Build history of the part. All positions in model axes, mm. A direction names the side the tool comes from. Coordinates: 2 decimals unless noted, no trailing zeros. Loops run counter-clockwise (first coordinate to the right, second up) from the corner with the lowest first, then second, coordinate; pieces in that order, holes last.
(1) Slice it at A-A (x = 0). Give the cut face in (y, z), and give its area (3 significant figures).
(2) Flat gauge pins, fed straight in: P1, Ø3, axis at y = 18, z = 8.5, coming from the -X side; P2, Ø18.5, axis at x = 0, y = 0, coming from the +Z side; P3, Ø7, axis at x = 0, y = -2.5, coming from the -Z side; P4, Ø8, axis at x = 0.5, y = 25, coming from the -Z side. Where does each tip first touch, or does it go through?
(3) Two-plate mould, pull along Y, no slides. Class faces 3 (the face through (-4.686, 35.694, 31.552)), 4 (the face through (7.8, -34.5, 64)), 5 (the face through (1.5, 11.4, 1.2)): pulls with the +Y half, pulls with the -Y half, needs draft (parallel to the pull), parting line crosses it, or undercut.
(4) Tool access for faces 1 (the face through (0, 0, 2.5)), 2 (the face through (-9, 9, 0)): list every direction of +Z, -Z, +X, -X, +Y, -Y with a clear straight run to the whole face (end or side of a thin tool).
(5) Slice it at D-D (z = 21). Give the cut face in (x, y), and give its area (3 significant figures).
(6) Wall check: L1, parallel to Y at x = 0, z = 1.65; L2, parallel to Y at x = 4, z = 49; L3, parallel to Y at x = -1, z = 26.5. Give the ranges that are in metal, low to high.
(7) Slice it at C-C (z = 52). Give the cut face in (x, y), and give its area (3 significant figures).
from build123d import *

# Parameters (mm, degrees)
SKETCH2_R           = 36
BOSS_EXTRUDE1_DEPTH = 74
CUT_REVOLVE1_ANGLE  = 180
CUT_EXTRUDE1_REACH  = 12
SKETCH5_W           = 97.630906447
SKETCH5_H           = 85.301230118
SKETCH6_R           = 11.5
CUT_EXTRUDE2_DEPTH  = 2.5


with BuildPart() as part:
    # Sketch2 → Boss-Extrude1 (new body)
    with BuildSketch(Plane.XY):
        Circle(SKETCH2_R)
    extrude(amount=BOSS_EXTRUDE1_DEPTH)

    # Sketch4 → Cut-Revolve1 (revolve, cut)
    with BuildSketch(Plane.XY.offset(69)):
        with BuildLine():
            Line((-35.5, 0), (35.5, 0))
            ThreePointArc((35.5, 0), (0, 35.5), (-35.5, 0))
        make_face()
    revolve(axis=Axis((-35.5, 0, 69), (-1, 0, 0)), revolution_arc=CUT_REVOLVE1_ANGLE, mode=Mode.SUBTRACT)

    # Sketch5 → Cut-Extrude1 (cut, up to next)
    with BuildSketch(Plane.XY.offset(64), mode=Mode.PRIVATE) as cut_extrude1_sk1:
        with Locations((-1.59772985, 0.365427289)):
            Rectangle(SKETCH5_W, SKETCH5_H)
    cut_extrude1_tool1 = extrude(cut_extrude1_sk1.sketch, amount=CUT_EXTRUDE1_REACH, mode=Mode.PRIVATE) & part.part
    add(cut_extrude1_tool1.solids().sort_by_distance((-1.59773, 0.365427, 64))[0], mode=Mode.SUBTRACT)

    # Sketch6 → Cut-Extrude2 (cut)
    with BuildSketch(Plane(origin=(0, 0, 0), x_dir=(-1, 0, 0), z_dir=(0, 0, -1))):
        Circle(SKETCH6_R)
    extrude(amount=-CUT_EXTRUDE2_DEPTH, mode=Mode.SUBTRACT)


solid = part.part
Response values:
1. outline: (-36, 0) - (-11.5, 0) - (-11.5, 2.5) - (11.5, 2.5) - (11.5, 0) - (36, 0) - (36, 64) - (35.15, 64) arc R35.5 cw to (-35.15, 64) - (-36, 64) - close
1. area: 2,920 mm2
2. P1: stops at x = -32
2. P2: stops at z = 34.73
2. P3: stops at z = 2.5
2. P4: stops at z = 0
3. face 3: parting line crosses it
3. face 4: needs draft
3. face 5: undercut
4. face 1: -Z
4. face 2: -Z, +X, -X, +Y, -Y
5. outline: circle Ø72 at (0, 0)
5. area: 4,070 mm2
6. L1: y = -36 to -11.5, 11.5 to 36
6. L2: y = -35.78 to -29.06, 29.06 to 35.78
6. L3: y = -35.99 to 35.99
7. outline: circle Ø72 at (0, 0); hole circle Ø62.33 at (0, 0)
7. area: 1,020 mm2
